```python
from build123d import *

# Parameters (mm, degrees)
SKETCH2_W           = 228.6
SKETCH2_H           = 228.6
BOSS_EXTRUDE2_DEPTH = 3.43
SKETCH3_R           = 45
CUT_EXTRUDE1_DEPTH  = 3.43
SKETCH4_R           = 2.6
CUT_EXTRUDE2_DEPTH  = 3.43
SKETCH4_3_R         = 2.6
CUT_EXTRUDE3_DEPTH  = 3.43
SKETCH4_4_R         = 2.6
CUT_EXTRUDE4_DEPTH  = 3.43
SKETCH13_W          = 63.6
SKETCH13_H          = 39.1
CUT_EXTRUDE6_DEPTH  = 10
SKETCH21_R          = 1.85
CUT_EXTRUDE11_DEPTH = 10
SKETCH16_R          = 1.8
CUT_EXTRUDE9_DEPTH  = 10
SKETCH17_R          = 1.73
SKETCH17_R_2        = 7.82641692
CUT_EXTRUDE10_DEPTH = 10


with BuildPart() as part:
    # Sketch2 → Boss-Extrude2 (new body)
    with BuildSketch(Plane(origin=(0, 0, 0), x_dir=(1, 0, 0), z_dir=(0, 1, 0))):
        Rectangle(SKETCH2_W, SKETCH2_H)
    extrude(amount=BOSS_EXTRUDE2_DEPTH)

    # Sketch3 → Cut-Extrude1 (cut)
    with BuildSketch(Plane(origin=(0, 3.43, 0), x_dir=(1, 0, 0), z_dir=(0, 1, 0))):
        with Locations(Location((-40.039608825, -44.823101489, 0), (0, 0, 270))):
            Circle(SKETCH3_R)
    extrude(amount=-CUT_EXTRUDE1_DEPTH, mode=Mode.SUBTRACT)

    # Sketch4 → Cut-Extrude2 (cut)
    with BuildSketch(Plane(origin=(0, 3.43, 0), x_dir=(1, 0, 0), z_dir=(0, 1, 0))):
        with Locations(Location((7.942522776, -1.692270962, 0), (0, 0, 270))):
            Circle(SKETCH4_R)
    extrude(amount=-CUT_EXTRUDE2_DEPTH, mode=Mode.SUBTRACT)

    # Sketch4_3 → Cut-Extrude3 (cut)
    with BuildSketch(Plane(origin=(0, 3.43, 0), x_dir=(1, 0, 0), z_dir=(0, 1, 0))):
        with Locations(Location((-87.581844281, 0, 0), (0, 0, 270))):
            Circle(SKETCH4_3_R)
    extrude(amount=-CUT_EXTRUDE3_DEPTH, mode=Mode.SUBTRACT)

    # Sketch4_4 → Cut-Extrude4 (cut)
    with BuildSketch(Plane(origin=(0, 3.43, 0), x_dir=(1, 0, 0), z_dir=(0, 1, 0))):
        with Locations(Location((7.942522776, -88.202101991, 0), (0, 0, 270))):
            Circle(SKETCH4_4_R)
        with Locations(Location((-87.581844281, -88.202101991, 0), (0, 0, 270))):
            Circle(SKETCH4_4_R)
    extrude(amount=-CUT_EXTRUDE4_DEPTH, mode=Mode.SUBTRACT)

    # Sketch13 → Cut-Extrude6 (cut)
    with BuildSketch(Plane(origin=(0, 3.43, 0), x_dir=(1, 0, 0), z_dir=(0, 1, 0))):
        with Locations((-25.511426019, 31.937893032)):
            Rectangle(SKETCH13_W, SKETCH13_H)
    extrude(amount=-CUT_EXTRUDE6_DEPTH, mode=Mode.SUBTRACT)

    # Sketch21 → Cut-Extrude11 (cut)
    with BuildSketch(Plane(origin=(0, 3.43, 0), x_dir=(1, 0, 0), z_dir=(0, 1, 0))):
        with Locations(Location((-80.511426019, 46.487893032, 0), (0, 0, 270))):
            Circle(SKETCH21_R)
        with Locations(Location((-68.861426019, 17.387893032, 0), (0, 0, 270))):
            Circle(SKETCH21_R)
        with Locations(Location((29.488573981, 17.387893032, 0), (0, 0, 270))):
            Circle(SKETCH21_R)
        with Locations(Location((17.838573981, 46.487893032, 0), (0, 0, 270))):
            Circle(SKETCH21_R)
    extrude(amount=-CUT_EXTRUDE11_DEPTH, mode=Mode.SUBTRACT)

    # Sketch16 → Cut-Extrude9 (cut)
    with BuildSketch(Plane(origin=(0, 3.43, 0), x_dir=(1, 0, 0), z_dir=(0, 1, 0))):
        with Locations(Location((99.249935188, -106.326440771, 0), (0, 0, 270))):
            Circle(SKETCH16_R)
        with Locations(Location((99.249935188, 100.705817131, 0), (0, 0, 270))):
            Circle(SKETCH16_R)
        with Locations(Location((-104.840818846, 100.705817131, 0), (0, 0, 270))):
            Circle(SKETCH16_R)
        with Locations(Location((-104.840818846, -106.326440771, 0), (0, 0, 270))):
            Circle(SKETCH16_R)
    extrude(amount=-CUT_EXTRUDE9_DEPTH, mode=Mode.SUBTRACT)

    # Sketch17 → Cut-Extrude10 (cut)
    with BuildSketch(Plane(origin=(0, 3.43, 0), x_dir=(1, 0, 0), z_dir=(0, 1, 0))):
        with Locations(Location((36.96258804, -19.846493577, 0), (0, 0, 270))):
            Circle(SKETCH17_R)
        with Locations(Location((36.676933631, -32.543280633, 0), (0, 0, 270))):
            Circle(SKETCH17_R)
        with Locations(Location((36.963684366, -44.799926749, 0), (0, 0, 270))):
            Circle(SKETCH17_R_2)
    extrude(amount=-CUT_EXTRUDE10_DEPTH, mode=Mode.SUBTRACT)


solid = part.part
```
Design review of the part built by this model. Coordinates are the model's own, in mm. Coordinates: 2 decimals unless noted, no trailing zeros. Loops run counter-clockwise (first coordinate to the right, second up) from the corner with the lowest first, then second, coordinate; pieces in that order, holes last. Notation, with made-up numbers: (-23.75, 18.5) - (35.25, 18.5) arc R15 cw to (35.25, 41.5) - close; hole circle Ø8 at (82, 22). An arc over 180 degrees is marked (long way). Use CSV: the item, a comma, the result in double quotes. Start each with the question number.
1) Wall thickness on L1, parallel to Z at x = -104.5, y = 2.7; L2, parallel to Z at x = -39, y = 0.9; L3, parallel to X at y = 0.85, z = -31: over which ranges is each line inside the solid? List them lowest first. Write a range as from..to.
2) Consider section C-C on z = 8. Write out the cut boundary in (x, y).
3) Consider section B-B on y = 2. Give the number of separate pieces and of enclosed holes in the cut face, then the cut area to 3 significant figures.
4) For pin 1 Ø4 at (x, z) = (36.68, 32.54) entering from -Y; pin 2 Ø2 at (x, z) = (36.96, 19.85) entering from -Y, all flat-tipped, find the tip position at first contact; note any pin that passes through.
5) The part is to be moulded in two halves that separate along X. For faces 1 (the cylindrical face through (8.057, 1.739, 85.605)), 2 (the flat face through (-2, 0, -2)), say which applies: +X half, -X half, draft (parallel to the pull), parting line (faces both ways), or undercut.
6) Consider section A-A on z = 58. Write out the cut boundary in (x, y).
Geometry says:
1,L1,"-114.3..-102.47, -98.94..104.56, 108.09..114.3"
1,L2,"-114.3..-51.49, -12.39..-0.16, 89.81..114.3"
1,L3,"-114.3..-57.31, 6.29..114.3"
2,outline,"(-114.3, 0) - (-65.91, 0) - (-65.91, 3.43) - (-114.3, 3.43) - close; (-14.17, 0) - (114.3, 0) - (114.3, 3.43) - (-14.17, 3.43) - close"
3,separate pieces,"1"
3,enclosed holes,"17"
3,area,"43,000 mm^2"
4,pin 1,"y = 0"
4,pin 2,"through"
5,face 1,"undercut"
5,face 2,"draft"
6,outline,"(-114.3, 0) - (-83.07, 0) - (-83.07, 3.43) - (-114.3, 3.43) - close; (2.99, 0) - (114.3, 0) - (114.3, 3.43) - (2.99, 3.43) - close"
